Autodesk Fusion 360 part; units mm, degrees
sketch "Sketch1" plane through (0, 0, 0) normal (0, 0, 1) x (1, 0, 0)
  line L0 (-47.25, 23.2) -> (47.25, 23.2)
  line L1 (47.25, 23.2) -> (47.25, -23.2)
  line L2 (47.25, -23.2) -> (-47.25, -23.2)
  line L3 (-47.25, -23.2) -> (-47.25, 23.2)
  line L4 (-47.25, 23.2) -> (47.25, -23.2) construction
  line L5 (47.25, 23.2) -> (-47.25, -23.2) construction
  dimension "d1" = 94.5
  dimension "d2" = 46.4
extrude "Extrude1" add sketch "Sketch1" along normal blind 2.5
sketch "Sketch2" plane through (0, 0, 2.5) normal (0, 0, 1) x (-1, 0, 0)
  line L0 (47.25, 23.2) -> (-47.25, 23.2)
  line L1 (-47.25, 23.2) -> (-47.25, -23.2)
  line L2 (-47.25, -23.2) -> (47.25, -23.2)
  line L3 (47.25, -23.2) -> (47.25, 23.2)
  line L4 (22.25, 6.7) -> (11.25, 6.7)
  line L5 (11.25, 6.7) -> (11.25, 23.2)
  line L6 (11.25, 23.2) -> (22.25, 23.2)
  line L7 (22.25, 23.2) -> (22.25, 6.7)
  line L8 (3.75, 1.7) -> (-7.25, 1.7)
  line L9 (-7.25, 1.7) -> (-7.25, 8.7)
  line L10 (-7.25, 8.7) -> (3.75, 8.7)
  line L11 (3.75, 8.7) -> (3.75, 1.7)
  dimension "d5" = 11
  dimension "d6" = 16.5
  dimension "d7" = 25
  dimension "d12" = 21.5
  dimension "d13" = 40
  dimension "d14" = 11
  dimension "d15" = 7
extrude "Extrude2" cut sketch "Sketch2" against normal blind 5 contours L0 L4 L5 L6 L7 | L8 L9 L10 L11
fillet "Fillet1" radius 2 2 edges at (-22.25, -6.7, 1.25) (-11.25, -6.7, 1.25)
fillet "Fillet2" radius 1 4 edges at (7.25, -1.7, 1.25) (-3.75, -1.7, 1.25) (-3.75, -8.7, 1.25) (7.25, -8.7, 1.25)
sketch "Sketch3" plane through (0, 0, 2.5) normal (0, 0, 1) x (-1, 0, 0)
  line L0 (11.25, 8.7) -> (11.25, 23.2)
  line L1 (11.25, 23.2) -> (-47.25, 23.2)
  line L2 (-47.25, 23.2) -> (-47.25, -23.2)
  line L3 (-47.25, -23.2) -> (47.25, -23.2)
  line L4 (47.25, -23.2) -> (47.25, 23.2)
  line L5 (47.25, 23.2) -> (22.25, 23.2)
  line L6 (22.25, 23.2) -> (22.25, 8.7)
  arc A0 (20.25, 6.7) -> (22.25, 8.7) centre (20.25, 8.7) ccw
  line L7 (20.25, 6.7) -> (13.25, 6.7)
  arc A1 (11.25, 8.7) -> (13.25, 6.7) centre (13.25, 8.7) ccw
  line L8 (-7.25, 2.7) -> (-7.25, 7.7)
  arc A2 (-6.25, 8.7) -> (-7.25, 7.7) centre (-6.25, 7.7) ccw
  line L9 (-6.25, 8.7) -> (2.75, 8.7)
  arc A3 (3.75, 7.7) -> (2.75, 8.7) centre (2.75, 7.7) ccw
  line L10 (3.75, 7.7) -> (3.75, 2.7)
  arc A4 (2.75, 1.7) -> (3.75, 2.7) centre (2.75, 2.7) ccw
  line L11 (2.75, 1.7) -> (-6.25, 1.7)
  arc A5 (-7.25, 2.7) -> (-6.25, 1.7) centre (-6.25, 2.7) ccw
  line L12 (-7.25, 5.2) -> (-7.25, 2.7)
equation "d2 = 52.65 mm - 6.25 mm"
Geometry check sheet. Reference: the model listing, model coordinates, mm. A direction names the side the tool comes from. Coordinates: 2 decimals unless noted, no trailing zeros. Order: outer loops, then holes, each group sorted by start corner. A loop starts at its lowest first (then second) coordinate and runs counter-clockwise, first axis right, second up. Notation, with made-up numbers: M -27.75,34.25 L -3.75,34.25 A28 cw -3.75,61.25 Z; hole C -36,41 d11. An arc over 180 degrees is marked long. Answer as a JSON object with one key per item and string values.
Q1. Cross-section at C-C on z = 0.7. Record the cut outline in (x, y), and give its area (3 significant figures).
Results are:
{"outline": "M -47.25,-23.2 L -22.25,-23.2 L -22.25,-8.7 A2 cw -20.25,-6.7 L -13.25,-6.7 A2 cw -11.25,-8.7 L -11.25,-23.2 L 47.25,-23.2 L 47.25,23.2 L -47.25,23.2 Z; hole M -3.75,-7.7 A1 ccw -2.75,-8.7 L 6.25,-8.7 A1 ccw 7.25,-7.7 L 7.25,-2.7 A1 ccw 6.25,-1.7 L -2.75,-1.7 A1 ccw -3.75,-2.7 Z", "area": "4,130 mm²"}
Q2. Scan lines: line 1 (X direction, y = -9.5, z = 1.6); line 2 (Y direction, x = 6, z = 0.15); line 3 (X direction, y = -3, z = 0.3). Record each from-to range of solid material in increasing order.
Results are:
{"line 1": "x = -47.25 to -22.25, -11.25 to 47.25", "line 2": "y = -23.2 to -8.7, -1.7 to 23.2", "line 3": "x = -47.25 to -3.75, 7.25 to 47.25"}
Q3. Release check for a two-part mould opening along Y. For faces 4 (the flat face through (2, -1.7, 1)), 5 (the cylindrical face through (-11.85, -7.27, 1.23)), 6 (the flat face through (-1, 0, 0)) record: released by +Y, released by -Y, zero draft, split by the parting line, or undercut.
Results are:
{"face 4": "undercut", "face 5": "released by -Y", "face 6": "zero draft"}
Q4. Cross-section at A-A on y = -19. Record the cut outline in (x, z), and give its area (3 significant figures).
Results are:
{"outline": "M -47.25,0 L -22.25,0 L -22.25,2.5 L -47.25,2.5 Z; M -11.25,0 L 47.25,0 L 47.25,2.5 L -11.25,2.5 Z", "area": "209 mm²"}
Q5. Cross-section at B-B on x = 2.5. Record the cut outline in (y, z), and give its area (3 significant figures).
Results are:
{"outline": "M -23.2,0 L -8.7,0 L -8.7,2.5 L -23.2,2.5 Z; M -1.7,0 L 23.2,0 L 23.2,2.5 L -1.7,2.5 Z", "area": "98.5 mm²"}
Q6. Tool access check on faces 1 (the flat face through (-22.25, -16, 1)), 2 (the flat face through (-3.75, -5, 1)), 3 (the flat face through (-47.25, 0, 1)). Record the directions out of +Z, -Z, +X, -X, +Y, -Y that give a thin tool (end or side, any length) a straight path to the whole face; none if there is none.
Results are:
{"face 1": "+Z, -Z, -Y", "face 2": "+Z, -Z", "face 3": "+Z, -Z, -X, +Y, -Y"}
